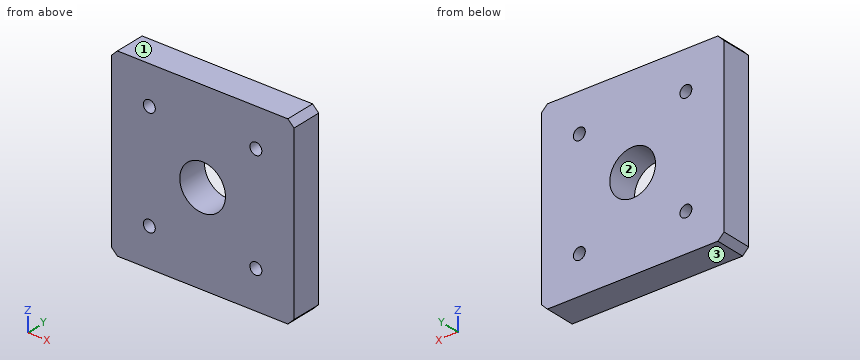
Autodesk Inventor part; units mm, degrees
ref_plane "YZ Plane" through (0, 0, 0) normal (1, 0, 0) x (0, 1, 0)
ref_plane "XZ Plane" through (0, 0, 0) normal (0, 1, 0) x (-1, 0, 0)
ref_plane "XY Plane" through (0, 0, 0) normal (0, 0, 1) x (1, 0, 0)
sketch "Sketch1" plane through (0, 0, 0) normal (0, 1, 0) x (-1, 0, 0)
  line L0 (-30, -30) -> (30, -30)
  line L1 (30, -30) -> (30, 30)
  line L2 (30, 30) -> (-30, 30)
  line L3 (-30, 30) -> (-30, -30)
  line L4 (-30, -30) -> (30, 30) construction
  line L5 (30, -30) -> (-30, 30) construction
  circle A0 centre (0, 0) radius 7.5
  dimension "d0" = 60
  dimension "d1" = 60
  dimension "d13" = 15
extrude "Extrusion1" add sketch "Sketch1" along normal blind 10
sketch "Sketch2" plane through (0, 10, 0) normal (0, 1, 0) x (1, 0, 0)
  line L0 (30, 30) -> (-30, 30)
  line L1 (-30, 30) -> (-30, -30)
  line L2 (-30, -30) -> (30, -30)
  line L3 (30, -30) -> (30, 30)
  line L4 (17.5, -17.5) -> (-17.5, -17.5)
  line L5 (-17.5, -17.5) -> (-17.5, 17.5)
  line L6 (-17.5, 17.5) -> (17.5, 17.5)
  line L7 (17.5, 17.5) -> (17.5, -17.5)
  line L8 (17.5, -17.5) -> (-17.5, 17.5) construction
  line L9 (-17.5, -17.5) -> (17.5, 17.5) construction
  line L10 (0, -17.5) -> (0, 17.5)
  line L11 (-17.5, 0) -> (17.5, 0)
  point P0 (0, 0)
  dimension "d4" = 35
  dimension "d5" = 35
hole "Hole1" at (-17.5, 10, 17.5) at (-17.5, 10, -17.5) at (17.5, 10, -17.5) at (17.5, 10, 17.5) direction (0, -1, 0) diameter 3.9 depth 10 tip angle 118
chamfer "Chamfer1" distance 2 angle 45 4 edges at (30, 5, 30) (30, 5, -30) (-30, 5, -30) (-30, 5, 30)
properties part number "00_XY_stage-CHUO_SEIKI_LD-647-R1-Top"
Source: CAD feature listing. Evaluate the final solid. Frame: model axes, mm. Face numbers are marked on the shaded views. Round coordinates to 2 decimals unless told otherwise and drop trailing zeros. Loops run counter-clockwise (first coordinate to the right, second up) from the corner with the lowest first, then second, coordinate; pieces in that order, holes last.
Q1. Section B-B, the plane x = 17.5. Return loops of the section in (y, z), plus the area to 3 significant figures.
Q2. First-contact query: P1, Ø3, axis at x = 17.5, z = 17.5, coming from the -Y side; P2, Ø3, axis at x = 13.5, z = 15, coming from the -Y side. Flat tips, straight axial feed; report the tip coordinate or a pass-through.
Q3. Section A-A, the plane z = 17.5. Return loops of the section in (x, y), plus the area to 3 significant figures.
Q4. Ray query, line 1 (X direction, y = 2, z = -17.5); line 2 (Z direction, x = 0, y = 3). Return the intervals inside material, ascending.
Q5. Section D-D, the plane y = 6. Return loops of the section in (x, z).
Q6. Section C-C, the plane x = 0. Return loops of the section in (y, z), plus the area to 3 significant figures.
Q7. Mould query, pull axis Z, two halves, no side actions, for the marked faces 1, 2 and 3. Classes: pulls with the +Z half, pulls with the -Z half, needs draft (parallel to the pull), parting line crosses it, or undercut.
Solutions:
1. outline: (0, -30) - (10, -30) - (10, -19.45) - (0, -19.45) - close; (0, -15.55) - (10, -15.55) - (10, 15.55) - (0, 15.55) - close; (0, 19.45) - (10, 19.45) - (10, 30) - (0, 30) - close
1. area: 522 mm2
2. P1: passes through
2. P2: stops at y = 0
3. outline: (-30, 0) - (-19.45, 0) - (-19.45, 10) - (-30, 10) - close; (-15.55, 0) - (15.55, 0) - (15.55, 10) - (-15.55, 10) - close; (19.45, 0) - (30, 0) - (30, 10) - (19.45, 10) - close
3. area: 522 mm2
4. line 1: x = -30 to -19.45, -15.55 to 15.55, 19.45 to 30
4. line 2: z = -30 to -7.5, 7.5 to 30
5. outline: (-30, -28) - (-28, -30) - (28, -30) - (30, -28) - (30, 28) - (28, 30) - (-28, 30) - (-30, 28) - close; hole circle Ø3.9 at (-17.5, -17.5); hole circle Ø3.9 at (-17.5, 17.5); hole circle Ø15 at (0, 0); hole circle Ø3.9 at (17.5, -17.5); hole circle Ø3.9 at (17.5, 17.5)
6. outline: (0, -30) - (10, -30) - (10, -7.5) - (0, -7.5) - close; (0, 7.5) - (10, 7.5) - (10, 30) - (0, 30) - close
6. area: 450 mm2
7. face 1: pulls with the +Z half
7. face 2: undercut
7. face 3: pulls with the -Z half
